```python
from build123d import *

# Parameters (mm, degrees)
SKETCH3_R           = 87.5
SKETCH3_R_2         = 77.5
BOSS_EXTRUDE1_DEPTH = 175
SKETCH3_2_R         = 77.5
BOSS_EXTRUDE2_DEPTH = 5
SKETCH4_R           = 25
CUT_EXTRUDE1_DEPTH  = 215.330352494


with BuildPart() as part:
    # Sketch3 → Boss-Extrude1 (new body)
    with BuildSketch(Plane(origin=(0, 0, 0), x_dir=(1, 0, 0), z_dir=(0, 1, 0))):
        with Locations(Location((0, 0, 0), (0, 0, 270))):
            Circle(SKETCH3_R)
        with Locations(Location((0, 0, 0), (0, 0, 270))):
            Circle(SKETCH3_R_2, mode=Mode.SUBTRACT)
    extrude(amount=BOSS_EXTRUDE1_DEPTH)

    # Sketch3_2 → Boss-Extrude2 (add)
    with BuildSketch(Plane(origin=(0, 0, 0), x_dir=(1, 0, 0), z_dir=(0, 1, 0))):
        with Locations(Location((0, 0, 0), (0, 0, 270))):
            Circle(SKETCH3_2_R)
    extrude(amount=BOSS_EXTRUDE2_DEPTH)

    # Sketch4 → Cut-Extrude1 (cut, through all)
    with BuildSketch(Plane(origin=(0, 0, 0), x_dir=(0, 0, -1), z_dir=(1, 0, 0))):
        with Locations((-47.5, 40)):
            Circle(SKETCH4_R)
    extrude(amount=-CUT_EXTRUDE1_DEPTH, mode=Mode.SUBTRACT)


solid = part.part
```
Model file for the job. Use its own axes, mm. A direction names the side the tool comes from. Coordinates: 2 decimals unless noted, no trailing zeros. Order: outer loops, then holes, each group sorted by start corner. A loop starts at its lowest first (then second) coordinate and runs counter-clockwise, first axis right, second up. Notation, with made-up numbers: (-12.75, 66) - (4.25, 66) arc R17 ccw to (4.25, 93) - close; hole circle Ø8 at (76, 16). An arc over 180 degrees is marked (long way). Return JSON: item names as keys, results as strings. Group by question number.
1) Tool access for faces 1 (the cylindrical face through (52.4, 88.8, -57.1)), 2 (the flat face through (-77.4, 175, -6.9)): list every direction of +Z, -Z, +X, -X, +Y, -Y with a clear straight run to the whole face (end or side of a thin tool).
2) Flat gauge pins, fed straight in: P1, Ø8, axis at x = -36, y = 65, coming from the -Z side; P2, Ø10, axis at y = 20.5, z = -9.5, coming from the -X side; P3, Ø8, axis at y = 129.5, z = 51.5, coming from the +X side. Where does each tip first touch, or does it go through?
3) Saw through at D-D, the plane x = -54. Write the cut outline in (y, z), plus the area to 3 significant figures.
4) Saw through at C-C, the plane z = 0. Write the cut outline in (x, y).
5) Probe line 1 (Y direction, x = -61.5, z = 47.5); line 2 (X direction, y = 109, z = 0). List the from-to ranges inside material, lowest first. Write a range as from..to.
6) Saw through at B-B, the plane x = 0. Write the cut outline in (y, z), plus the area to 4 significant figures.
7) Saw through at A-A, the plane z = 48.5. Write the cut outline in (x, y).
8) Mould opens along Y. For faces 3 (the flat face through (1, 5, -1)), 4 (the cylindrical face through (-55.84, 24.21, 66.88)), 5 (the flat face through (1, 0, -1)) say: released by +Y, released by -Y, zero draft, split by the parting line, or undercut.
Values found:
{
 "1": {"face 1": "+Y", "face 2": "+Z, -Z, +X, -X, +Y"},
 "2": {"P1": "stops at z = -81.44", "P2": "stops at x = -87.38", "P3": "stops at x = 73.48"},
 "3": {"outline": "(0, -68.85) - (175, -68.85) - (175, -55.59) - (5, -55.59) - (5, 55.59) - (16.35, 55.59) arc R25 cw to (26.99, 68.85) - (0, 68.85) - close; (53.01, 68.85) arc R25 cw to (63.65, 55.59) - (175, 55.59) - (175, 68.85) - close", "area": "4,680 mm²"},
 "4": {"outline": "(-87.5, 0) - (87.5, 0) - (87.5, 175) - (77.5, 175) - (77.5, 5) - (-77.5, 5) - (-77.5, 175) - (-87.5, 175) - close"},
 "5": {"line 1": "y = 0..15, 65..175", "line 2": "x = -87.5..-77.5, 77.5..87.5"},
 "6": {"outline": "(0, -87.5) - (175, -87.5) - (175, -77.5) - (5, -77.5) - (5, 77.5) - (175, 77.5) - (175, 87.5) - (0, 87.5) - close", "area": "4,275 mm²"},
 "7": {"outline": "(-72.83, 0) - (72.83, 0) - (72.83, 175) - (60.45, 175) - (60.45, 5) - (-60.45, 5) - (-60.45, 15.02) - (-72.83, 15.02) - close; (-72.83, 64.98) - (-60.45, 64.98) - (-60.45, 175) - (-72.83, 175) - close"},
 "8": {"face 3": "released by +Y", "face 4": "undercut", "face 5": "released by -Y"}
}
